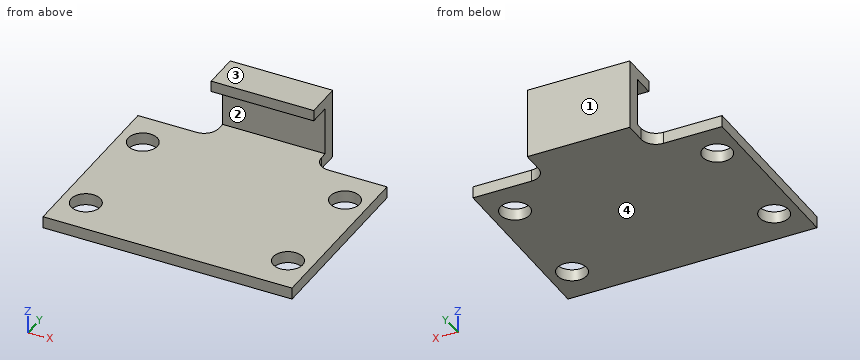
```python
from build123d import *

# Parameters (mm, degrees)
SKETCH1_W           = 43.18
SKETCH1_H           = 50.8
BOSS_EXTRUDE1_DEPTH = 2.032
SKETCH2_R           = 2.54
CUT_EXTRUDE1_DEPTH  = 34.397861069
SKETCH3_W           = 43.18
SKETCH3_H           = 2.54
BOSS_EXTRUDE2_DEPTH = 8.3185
SKETCH4_W           = 43.18
SKETCH4_H           = 6.35
BOSS_EXTRUDE3_DEPTH = 1.905
SKETCH5_W           = 12.2555
SKETCH5_H           = 6.35
CUT_EXTRUDE2_DEPTH  = 12.7
SKETCH6_W           = 12.2555
SKETCH6_H           = 6.35
CUT_EXTRUDE3_DEPTH  = 12.7
FILLET1_R           = 2.54
SKETCH7_W           = 43.18
SKETCH7_H           = 12.7
CUT_EXTRUDE4_DEPTH  = 12.7


with BuildPart() as part:
    # Sketch1 → Boss-Extrude1 (new body)
    with BuildSketch(Plane.XY):
        Rectangle(SKETCH1_W, SKETCH1_H)
    extrude(amount=BOSS_EXTRUDE1_DEPTH)

    # Sketch2 → Cut-Extrude1 (cut, through all)
    with BuildSketch(Plane.XY.offset(2.032)):
        with Locations((-17.526, 12.827)):
            Circle(SKETCH2_R)
        with Locations((-17.526, -6.223)):
            Circle(SKETCH2_R)
        with Locations(Location((17.526, -6.223, 0), (0, 0, 180))):
            Circle(SKETCH2_R)
        with Locations(Location((17.526, 12.827, 0), (0, 0, 180))):
            Circle(SKETCH2_R)
    extrude(amount=-CUT_EXTRUDE1_DEPTH, mode=Mode.SUBTRACT)

    # Sketch3 → Boss-Extrude2 (add)
    with BuildSketch(Plane.XY.offset(2.032)):
        with Locations((0, 24.13)):
            Rectangle(SKETCH3_W, SKETCH3_H)
    extrude(amount=BOSS_EXTRUDE2_DEPTH)

    # Sketch4 → Boss-Extrude3 (add)
    with BuildSketch(Plane.XY.offset(10.3505)):
        with Locations((0, 22.225)):
            Rectangle(SKETCH4_W, SKETCH4_H)
    extrude(amount=BOSS_EXTRUDE3_DEPTH)

    # Sketch5 → Cut-Extrude2 (cut)
    with BuildSketch(Plane(origin=(21.59, 0, 0), x_dir=(0, 0, -1), z_dir=(1, 0, 0))):
        with Locations((-6.12775, 22.225)):
            Rectangle(SKETCH5_W, SKETCH5_H)
    extrude(amount=-CUT_EXTRUDE2_DEPTH, mode=Mode.SUBTRACT)

    # Sketch6 → Cut-Extrude3 (cut)
    with BuildSketch(Plane.ZY.offset(21.59)):
        with Locations((6.12775, 22.225)):
            Rectangle(SKETCH6_W, SKETCH6_H)
    extrude(amount=-CUT_EXTRUDE3_DEPTH, mode=Mode.SUBTRACT)

    # Fillet1
    fillet1_edges = [part.edges().sort_by_distance(p)[0] for p in [
        (8.89, 19.05, 1.016),
        (-8.89, 19.05, 1.016),
    ]]
    fillet(fillet1_edges, radius=FILLET1_R)

    # Sketch7 → Cut-Extrude4 (cut)
    with BuildSketch(Plane.XY.offset(2.032)):
        with Locations((0, -19.05)):
            Rectangle(SKETCH7_W, SKETCH7_H)
    extrude(amount=-CUT_EXTRUDE4_DEPTH, mode=Mode.SUBTRACT)


solid = part.part
```
For this review, take the finished solid that the model builds, in its own axes (mm). Face numbers are marked on the shaded views. Round coordinates to 2 decimals unless told otherwise and drop trailing zeros. Loops run counter-clockwise (first coordinate to the right, second up) from the corner with the lowest first, then second, coordinate; pieces in that order, holes last.
(1) We need section A-A (x = -16.5). Give the boundary of the cut face in (y, z).
Returned:
outline: (-12.7, 0) - (-8.55, 0) - (-8.55, 2.03) - (-12.7, 2.03) - close; (-3.9, 0) - (10.5, 0) - (10.5, 2.03) - (-3.9, 2.03) - close; (15.15, 0) - (19.05, 0) - (19.05, 2.03) - (15.15, 2.03) - close
(2) We need section D-D (z = 4.5). Give the boundary of the cut face in (x, y), plus the area to 3 significant figures.
Returned:
outline: (-8.89, 22.86) - (8.89, 22.86) - (8.89, 25.4) - (-8.89, 25.4) - close
area: 45.2 mm2
(3) Mouldability with a two-part tool opening along Z and no side actions: class the marked faces 1, 2, 3 and 4 as released by +Z, released by -Z, zero draft, split by the parting line, or undercut.
Returned:
face 1: zero draft
face 2: undercut
face 3: released by +Z
face 4: released by -Z
(4) Clearance check with flat-ended pins moving along their axes: P1, Ø5, axis at y = 21, z = 7.5, coming from the +X side; P2, Ø1.5, axis at x = -2, y = 12, coming from the +Z side; P3, Ø4, axis at y = 21, z = 3.5, coming from the -X side; P4, Ø4, axis at x = 17.526, y = -6.223, coming from the +Z side. State where each tip first meets the part, or that it passes through.
Returned:
P1: stops at x = 8.89
P2: stops at z = 2.03
P3: stops at x = -9.8
P4: passes through
(5) We need section B-B (x = 5.5). Give the boundary of the cut face in (y, z), plus the area to 3 significant figures.
Returned:
outline: (-12.7, 0) - (25.4, 0) - (25.4, 12.26) - (19.05, 12.26) - (19.05, 10.35) - (22.86, 10.35) - (22.86, 2.03) - (-12.7, 2.03) - close
area: 111 mm2
(6) Wall thickness on line 1 along Z through (x, y) = (-6.5, 17.5); line 2 along Y through (x, z) = (-8.5, 9); line 3 along Y through (x, z) = (4, 11.5): over which ranges is each line inside the solid? List them lowest first.
Returned:
line 1: z = 0 to 2.03
line 2: y = 22.86 to 25.4
line 3: y = 19.05 to 25.4
(7) We need section C-C (y = 23.5). Give the boundary of the cut face in (x, z).
Returned:
outline: (-8.89, 0) - (8.89, 0) - (8.89, 12.26) - (-8.89, 12.26) - close
